Work out the finished part from the listing and answer in its coordinate system (mm). Face numbers are marked on the shaded views. A direction names the side the tool comes from. Coordinates: 2 decimals unless noted, no trailing zeros. Write each loop counter-clockwise with the first axis right and the second up, starting at its lowest first coordinate (ties: lowest second). Pieces come first, ordered by that corner, then holes. Notation, with made-up numbers: M 39.5,69.5 L 82.5,69.5 A32 cw 82.5,99.5 Z; hole C -33.5,77 d7. An arc over 180 degrees is marked long. Use CSV: the item, a comma, the result in double quotes.
from build123d import *

# Parameters (mm, degrees)
SKETCH1_R                = 31
SKETCH1_R_2              = 7
BOSS_EXTRUDE1_DEPTH      = 8.25
CUT_EXTRUDE1_DEPTH       = 9.25
FILLET1_R                = 1
CIRPATTERN2_COUNT        = 5
FILLET1_OF_CIRPATTERN2_R = 1
CUT_EXTRUDE2_DEPTH       = 1.8
CIRPATTERN3_COUNT        = 5
CIRPATTERN3_COPY_1_DEPTH = 1.8
CIRPATTERN3_COPY_2_DEPTH = 1.8
CIRPATTERN3_COPY_3_DEPTH = 1.8
CIRPATTERN3_COPY_4_DEPTH = 1.8
SKETCH5_R                = 2.75
CUT_EXTRUDE4_DEPTH       = 9.25
CIRPATTERN4_COUNT        = 5
SKETCH8_R                = 3.5
BOSS_EXTRUDE2_DEPTH      = 3.75
SKETCH9_R                = 2
CUT_EXTRUDE6_DEPTH       = 4
SKETCH10_R               = 1.5
BOSS_EXTRUDE3_DEPTH      = 4
CIRPATTERN6_COUNT        = 5


with BuildPart() as part:
    # Sketch1 → Boss-Extrude1 (new body)
    with BuildSketch(Plane(origin=(0, 0, 0), x_dir=(1, 0, 0), z_dir=(0, 1, 0))):
        Circle(SKETCH1_R)
        Circle(SKETCH1_R_2, mode=Mode.SUBTRACT)
    extrude(amount=BOSS_EXTRUDE1_DEPTH)

    # Sketch2 → Cut-Extrude1 (cut, through all)
    with BuildSketch(Plane.XZ):
        with BuildLine():
            Line((-10, -29.342801502), (-10, -20.028684822))
            ThreePointArc((-10, -20.028684822), (0, -18.25), (10, -20.028684822))
            Line((10, -20.028684822), (10, -29.342801502))
            ThreePointArc((10, -29.342801502), (0, -31), (-10, -29.342801502))
        make_face()
    cut_extrude1 = extrude(amount=-CUT_EXTRUDE1_DEPTH, mode=Mode.SUBTRACT)

    # Fillet1
    fillet1_edges = [part.edges().sort_by_distance(p)[0] for p in [
        (-10, 4.125, -20.028684822),
        (10, 4.125, -20.028684822),
    ]]
    fillet(fillet1_edges, radius=FILLET1_R)

    # CirPattern2: Cut-Extrude1 ×5 about axis
    cirpattern2_axis = Axis((0, 0, 0), (0, 1, 0))
    for i in range(1, CIRPATTERN2_COUNT):
        add(cut_extrude1.rotate(cirpattern2_axis, i * 360 / CIRPATTERN2_COUNT), mode=Mode.SUBTRACT)

    # Fillet1 of CirPattern2
    fillet1_of_cirpattern2_edges = [part.edges().sort_by_distance(p)[0] for p in [
        (-22.138581157, 4.125, 3.321361178),
        (-15.958241269, 4.125, -15.699769148),
        (-3.682395618, 4.125, 22.081398919),
        (-19.862735505, 4.125, 10.325693873),
        (19.862735505, 4.125, 10.325693873),
        (3.682395618, 4.125, 22.081398919),
        (15.958241269, 4.125, -15.699769148),
        (22.138581157, 4.125, 3.321361178),
    ]]
    fillet(fillet1_of_cirpattern2_edges, radius=FILLET1_OF_CIRPATTERN2_R)

    # Sketch3 → Cut-Extrude2 (cut)
    with BuildSketch(Plane.ZY.offset(-10)):
        Polygon((-27.6, 8.25), (-24.4, 8.25), (-24.4, 7.05), (-24.8, 6.65), (-27.2, 6.65), (-27.6, 7.05), align=None)
    cut_extrude2 = extrude(amount=-CUT_EXTRUDE2_DEPTH, mode=Mode.SUBTRACT)

    # Mirror1: Cut-Extrude2 across plane
    add(cut_extrude2.mirror(Plane(origin=(0, 0, 0), x_dir=(0, 0, 1), z_dir=(1, 0, 0))), mode=Mode.SUBTRACT)

    # CirPattern3: Cut-Extrude2 ×5 about axis
    cirpattern3_axis = Axis((0, 0, 0), (0, 1, 0))
    for i in range(1, CIRPATTERN3_COUNT):
        add(cut_extrude2.rotate(cirpattern3_axis, i * 360 / CIRPATTERN3_COUNT), mode=Mode.SUBTRACT)

    # CirPattern3 copy 1 sketch → CirPattern3 copy 1 (cut)
    with BuildSketch(Plane(origin=(-3.090169944, 0, 9.510565163), x_dir=(0.951056516, 0, 0.309016994), z_dir=(0.309016994, 0, -0.951056516))):
        Polygon((-27.6, -8.25), (-24.4, -8.25), (-24.4, -7.05), (-24.8, -6.65), (-27.2, -6.65), (-27.6, -7.05), align=None)
    extrude(amount=-CIRPATTERN3_COPY_1_DEPTH, mode=Mode.SUBTRACT)

    # CirPattern3 copy 2 sketch → CirPattern3 copy 2 (cut)
    with BuildSketch(Plane(origin=(8.090169944, 0, 5.877852523), x_dir=(0.587785252, 0, -0.809016994), z_dir=(-0.809016994, 0, -0.587785252))):
        Polygon((-27.6, -8.25), (-24.4, -8.25), (-24.4, -7.05), (-24.8, -6.65), (-27.2, -6.65), (-27.6, -7.05), align=None)
    extrude(amount=-CIRPATTERN3_COPY_2_DEPTH, mode=Mode.SUBTRACT)

    # CirPattern3 copy 3 sketch → CirPattern3 copy 3 (cut)
    with BuildSketch(Plane(origin=(8.090169944, 0, -5.877852523), x_dir=(-0.587785252, 0, -0.809016994), z_dir=(-0.809016994, 0, 0.587785252))):
        Polygon((-27.6, -8.25), (-24.4, -8.25), (-24.4, -7.05), (-24.8, -6.65), (-27.2, -6.65), (-27.6, -7.05), align=None)
    extrude(amount=-CIRPATTERN3_COPY_3_DEPTH, mode=Mode.SUBTRACT)

    # CirPattern3 copy 4 sketch → CirPattern3 copy 4 (cut)
    with BuildSketch(Plane(origin=(-3.090169944, 0, -9.510565163), x_dir=(-0.951056516, 0, 0.309016994), z_dir=(0.309016994, 0, 0.951056516))):
        Polygon((-27.6, -8.25), (-24.4, -8.25), (-24.4, -7.05), (-24.8, -6.65), (-27.2, -6.65), (-27.6, -7.05), align=None)
    extrude(amount=-CIRPATTERN3_COPY_4_DEPTH, mode=Mode.SUBTRACT)

    # Sketch5 → Cut-Extrude4 (cut, through all)
    with BuildSketch(Plane.XZ):
        with Locations((0, 26)):
            Circle(SKETCH5_R)
    cut_extrude4 = extrude(amount=-CUT_EXTRUDE4_DEPTH, mode=Mode.SUBTRACT)

    # CirPattern4: Cut-Extrude4 ×5 about axis
    cirpattern4_axis = Axis((0, 0, 0), (0, 1, 0))
    for i in range(1, CIRPATTERN4_COUNT):
        add(cut_extrude4.rotate(cirpattern4_axis, i * 360 / CIRPATTERN4_COUNT), mode=Mode.SUBTRACT)

    # Sketch8 → Boss-Extrude2 (add)
    with BuildSketch(Plane.XZ):
        with Locations((0, -12.5)):
            Circle(SKETCH8_R)
    boss_extrude2 = extrude(amount=BOSS_EXTRUDE2_DEPTH)

    # Sketch9 → Cut-Extrude6 (cut)
    with BuildSketch(Plane.XZ):
        with Locations((0, 12.5)):
            Circle(SKETCH9_R)
    cut_extrude6 = extrude(amount=-CUT_EXTRUDE6_DEPTH, mode=Mode.SUBTRACT)

    # Sketch10 → Boss-Extrude3 (add)
    with BuildSketch(Plane.XZ.offset(3.75)):
        with Locations((0, -12.5)):
            Circle(SKETCH10_R)
    boss_extrude3 = extrude(amount=BOSS_EXTRUDE3_DEPTH)

    # CirPattern6: Boss-Extrude2, Cut-Extrude6, Boss-Extrude3 ×5 about axis
    cirpattern6_axis = Axis((0, 0, 0), (0, 1, 0))
    for i in range(1, CIRPATTERN6_COUNT):
        add(boss_extrude2.rotate(cirpattern6_axis, i * 360 / CIRPATTERN6_COUNT))
        add(cut_extrude6.rotate(cirpattern6_axis, i * 360 / CIRPATTERN6_COUNT), mode=Mode.SUBTRACT)
        add(boss_extrude3.rotate(cirpattern6_axis, i * 360 / CIRPATTERN6_COUNT))


solid = part.part
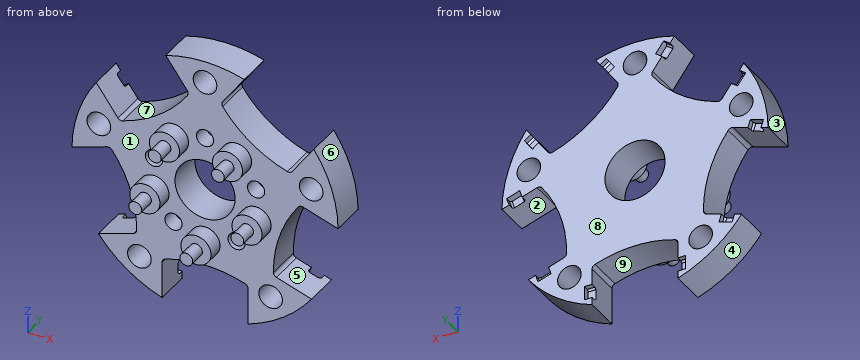
Item 1: For a pull along Z with two mould halves and no side action, classify the marked faces 6, 7, 8 and 9 as released by +Z, released by -Z, zero draft, split by the parting line, or undercut.
Answer:
face 6,"released by +Z"
face 7,"undercut"
face 8,"zero draft"
face 9,"released by -Z"
Item 2: The part is cut by section B-B (z = -4). Write down the section's boundary in (x, y), then the cut area to 3 significant figures.
Answer:
outline,"M -17.94,0 L -15.39,0 L -15.39,-3.75 L -13.38,-3.75 L -13.38,-7.75 L -10.39,-7.75 L -10.39,-3.75 L -8.39,-3.75 L -8.39,0 L -5.74,0 L -5.74,8.25 L -17.94,8.25 Z; M 5.74,0 L 8.39,0 L 8.39,-3.75 L 10.39,-3.75 L 10.39,-7.75 L 13.38,-7.75 L 13.38,-3.75 L 15.39,-3.75 L 15.39,0 L 17.94,0 L 17.94,8.25 L 5.74,8.25 Z"
area,"278 mm2"
Item 3: A tool of negligible diameter and unlimited length cuts with its end or side. For the marked faces 1, 2, 3, 4 and 5, from which of +Z, -Z, +X, -X, +Y, -Y can it reach the whole face along a straight path? Write none if from no direction.
Answer:
face 1,"-Y"
face 2,"+Y, -Y"
face 3,"+Z, -X, +Y, -Y"
face 4,"-Z, -X, +Y, -Y"
face 5,"+X, +Y, -Y"
Item 4: The part is cut by section A-A (x = 0). Write down the section's boundary in (y, z), then the cut area to 3 significant figures.
Answer:
outline,"M -7.75,-14 L -3.75,-14 L -3.75,-16 L 0,-16 L 0,-18.25 L 8.25,-18.25 L 8.25,-7 L 0,-7 L 0,-9 L -3.75,-9 L -3.75,-11 L -7.75,-11 Z; M 0,7 L 8.25,7 L 8.25,23.25 L 0,23.25 L 0,14.5 L 4,14.5 L 4,10.5 L 0,10.5 Z; M 0,28.75 L 8.25,28.75 L 8.25,31 L 0,31 Z"
area,"268 mm2"
Item 5: Given pin 1 (5 mm diameter, centred on x = -11.89, z = 3.86, fed in from -Y); pin 2 (1.5 mm diameter, centred on x = 14, z = -5.5, fed in from -Y); pin 3 (2 mm diameter, centred on y = 5.5, z = -4.5, fed in from -X); pin 4 (5 mm diameter, centred on x = 15.28, z = -21.03, fed in from +Y), each flat-ended and moving along its own axis, determine where each tip first touches the part or whether it passes through.
Answer:
pin 1,"stops at y = 0"
pin 2,"stops at y = -3.75"
pin 3,"stops at x = -18.15"
pin 4,"passes through"
Item 6: The part is cut by section C-C (y = 5.5). Count the separate pieces of the cut face and the enclosed holes in it, then the cut area to 3 significant figures.
Answer:
separate pieces,"1"
enclosed holes,"6"
area,"1,590 mm2"
Item 7: Consider probe 1 along Z at (x, y) = (24, 2); probe 2 along X at (y, z) = (2.5, -11.5); probe 3 along Z at (x, y) = (19, 3.25). Determine where each line is inside the solid, lowest interval first.
Answer:
probe 1,"z = -19.62 to -18.31, 2.72 to 5.38, 10.69 to 16.02"
probe 2,"x = -16.1 to -8.79, -5.91 to 5.91, 8.79 to 16.1"
probe 3,"z = -24.49 to -16.69, -1.63 to 10.58"
